Verification items for the finished model (mm, model axes). A direction names the side the tool comes from. Give positions to 0.01 mm unless a question says otherwise; leave off trailing zeros. Loops run counter-clockwise (first coordinate to the right, second up) from the corner with the lowest first, then second, coordinate; pieces in that order, holes last. Notation, with made-up numbers: (47.5, 6.25) -> (104.5, 6.25) arc R32 ccw to (104.5, 36.25) -> close; hole circle Ø11 at (-36.5, 61). An arc over 180 degrees is marked (long way). Answer in a Markdown table with one row per item. Add a question column.
Q1. Section check B-B on z = 51. Enter the section's corners in (x, y).
Q2. Section check C-C on y = 27. Enter the section's corners in (x, z), and give its area (3 significant figures).
Q3. Material ranges on probe 1 along Y at (x, z) = (-12, 32.5); probe 2 along Z at (x, y) = (-13, 5), recorded low to high.
Q4. Release check for a two-part mould opening along X. For faces 1 (the face through (50, -1, 51)), 2 (the face through (-50, -1, 51)), 3 (the face through (-1, -50, 51)), 4 (the face through (-1, -48.5, 54)) record: pulls with the +X half, pulls with the -X half, needs draft (parallel to the pull), parting line crosses it, or undercut.
Q5. Section check A-A on x = -10.5. Enter the section's corners in (y, z), and give its area (3 significant figures).
Q6. Set-up check for faces 5 (the face through (-1, 48.5, 54)), 6 (the face through (-1, -1, 0)): record each of +Z, -Z, +X, -X, +Y, -Y from which the full face is reachable in a straight line by a thin tool's end or side.
Q7. Gauge pin test, flat ends, axial feed: P1, Ø12, axis at x = -10.5, y = -38.5, coming from the +Z side; P2, Ø1.2, axis at x = -38.44, z = 4.57, coming from the -Y side. Record the tip position at first contact, or that the pin passes through.
```python
from build123d import *

# Parameters (mm, degrees)
SKETCH1_W           = 100
SKETCH1_H           = 100
BOSS_EXTRUDE1_DEPTH = 3
SKETCH4_W           = 100
SKETCH4_H           = 100
BOSS_EXTRUDE2_DEPTH = 100
SKETCH5_W           = 97
SKETCH5_H           = 97
CUT_EXTRUDE1_DEPTH  = 100
SKETCH6_R           = 1
CUT_EXTRUDE2_DEPTH  = 3
SKETCH7_W           = 18.8
SKETCH7_H           = 13.7
CUT_EXTRUDE3_DEPTH  = 3
CUT_EXTRUDE4_DEPTH  = 3


with BuildPart() as part:
    # Sketch1 → Boss-Extrude1 (new body)
    with BuildSketch(Plane(origin=(0, 0, 0), x_dir=(0, 1, 0), z_dir=(0, 0, 1))):
        Rectangle(SKETCH1_W, SKETCH1_H)
    extrude(amount=BOSS_EXTRUDE1_DEPTH)

    # Sketch4 → Boss-Extrude2 (add)
    with BuildSketch(Plane.XY.offset(3)):
        Rectangle(SKETCH4_W, SKETCH4_H)
    extrude(amount=BOSS_EXTRUDE2_DEPTH)

    # Sketch5 → Cut-Extrude1 (cut)
    with BuildSketch(Plane.XY.offset(103)):
        Rectangle(SKETCH5_W, SKETCH5_H)
    extrude(amount=-CUT_EXTRUDE1_DEPTH, mode=Mode.SUBTRACT)

    # Sketch6 → Cut-Extrude2 (cut)
    with BuildSketch(Plane.XZ.offset(50)):
        with Locations(Location((-45.693823315, 4.571208487, 0), (0, 0, 270))):
            Circle(SKETCH6_R)
        with Locations(Location((-38.438385154, 4.571208487, 0), (0, 0, 270))):
            Circle(SKETCH6_R)
        with Locations(Location((-29.79360777, 4.571208487, 0), (0, 0, 270))):
            Circle(SKETCH6_R)
    extrude(amount=-CUT_EXTRUDE2_DEPTH, mode=Mode.SUBTRACT)

    # Sketch7 → Cut-Extrude3 (cut)
    with BuildSketch(Plane.XZ.offset(50)):
        with Locations((-3.258424026, 11.15)):
            Rectangle(SKETCH7_W, SKETCH7_H)
    extrude(amount=-CUT_EXTRUDE3_DEPTH, mode=Mode.SUBTRACT)

    # Sketch8 → Cut-Extrude4 (cut)
    with BuildSketch(Plane.XZ.offset(50)):
        with BuildLine():
            Line((19.795752189, 9), (26.855752189, 9))
            ThreePointArc((26.855752189, 9), (28.135752189, 7.72), (26.855752189, 6.44))
            Line((26.855752189, 6.44), (19.795752189, 6.44))
            ThreePointArc((19.795752189, 6.44), (18.515752189, 7.72), (19.795752189, 9))
        make_face()
    extrude(amount=-CUT_EXTRUDE4_DEPTH, mode=Mode.SUBTRACT)


solid = part.part
```
Taken from the geometry:
| question | item | result |
|---|---|---|
| 1 | outline | (-50, -50) -> (50, -50) -> (50, 50) -> (-50, 50) -> close; hole (-48.5, -48.5) -> (48.5, -48.5) -> (48.5, 48.5) -> (-48.5, 48.5) -> close |
| 2 | outline | (-50, 0) -> (50, 0) -> (50, 103) -> (48.5, 103) -> (48.5, 3) -> (-48.5, 3) -> (-48.5, 103) -> (-50, 103) -> close |
| 2 | area | 600 mm² |
| 3 | probe 1 | y = -50 to -48.5, 48.5 to 50 |
| 3 | probe 2 | z = 0 to 3 |
| 4 | face 1 | pulls with the +X half |
| 4 | face 2 | pulls with the -X half |
| 4 | face 3 | needs draft |
| 4 | face 4 | undercut |
| 5 | outline | (-50, 0) -> (50, 0) -> (50, 103) -> (48.5, 103) -> (48.5, 3) -> (-48.5, 3) -> (-48.5, 4.3) -> (-50, 4.3) -> close; (-50, 18) -> (-48.5, 18) -> (-48.5, 103) -> (-50, 103) -> close |
| 5 | area | 579 mm² |
| 6 | face 5 | +Z |
| 6 | face 6 | -Z, +X, -X, +Y, -Y |
| 7 | P1 | stops at z = 3 |
| 7 | P2 | stops at y = 48.5 |
